from build123d import *

# Parameters (mm, degrees)
Y_KSEKLIK_EKSTR_ZYON3_DEPTH = 76
IZIM9_W                     = 50
IZIM9_H                     = 50
KES_EKSTR_ZYON2_DEPTH       = 72
RADYUS2_RADIUS              = 38
RADYUS2_LENGTH              = 18
IZIM10_R                    = 12.5
KES_EKSTR_ZYON3_DEPTH       = 260.686142434
FEDER1_REACH                = 253.207
IZIM11_WALL_W               = 579.380403386
IZIM11_WALL_H               = 22


with BuildPart() as part:
    # Çizim8 → Yükseklik-Ekstrüzyon3 (new body)
    with BuildSketch(Plane.XY):
        Polygon((-185.934081036, 55.935614824), (-109.934081036, 55.935614824), (-109.934081036, -16.064385176), (-241.934081036, -16.064385176), (-241.934081036, 1.935614824), (-185.934081036, 1.935614824), align=None)
    extrude(amount=Y_KSEKLIK_EKSTR_ZYON3_DEPTH)

    # Çizim9 → Kes-Ekstrüzyon2 (cut)
    with BuildSketch(Plane(origin=(0, 55.935614824, 0), x_dir=(1, 0, 0), z_dir=(0, 1, 0))):
        with Locations((-147.934081036, -38)):
            Rectangle(IZIM9_W, IZIM9_H)
    extrude(amount=-KES_EKSTR_ZYON2_DEPTH, mode=Mode.SUBTRACT)

    # Radyus2: full round fillet: the end face becomes a half cylinder, R = half its width
    radyus2_face = Plane((-241.934081036, -7.064385176, 38), x_dir=(0, 1, 0), z_dir=(-1, 0, 0))  # on the end face: x along it, z out of the body
    radyus2_slab = radyus2_face.offset(-RADYUS2_RADIUS / 2) * Box(RADYUS2_LENGTH, 2 * RADYUS2_RADIUS, RADYUS2_RADIUS, mode=Mode.PRIVATE)  # the body's end, R deep
    radyus2_round = Plane((-203.934081036, -7.064385176, 38), x_dir=(-1, 0, 0), z_dir=(0, 1, 0)) * Cylinder(RADYUS2_RADIUS, RADYUS2_LENGTH, mode=Mode.PRIVATE)  # its axis R under the face
    add(radyus2_slab - radyus2_round, mode=Mode.SUBTRACT)

    # Çizim10 → Kes-Ekstrüzyon3 (cut, through all)
    with BuildSketch(Plane.XY.offset(76)):
        with Locations((-147.934081036, 19.935614824)):
            Circle(IZIM10_R)
    extrude(amount=-KES_EKSTR_ZYON3_DEPTH, mode=Mode.SUBTRACT)

    # Çizim11 wall → Feder1 (add, up to next)
    with BuildSketch(Plane(origin=(-211.934081036, 28.935614824, 38), x_dir=(-0.693641687066, -0.720320213491, 0), z_dir=(0.720320213491, -0.693641687066, 0)), mode=Mode.PRIVATE) as feder1_sk1:
        Rectangle(IZIM11_WALL_W, IZIM11_WALL_H)
    feder1_tool1 = extrude(feder1_sk1.sketch, amount=FEDER1_REACH, mode=Mode.PRIVATE) - part.part
    add(feder1_tool1.solids().sort_by_distance((-211.934081036, 28.935614824, 38))[0])


solid = part.part
CAD build for the part. Positions are in the model's coordinates, mm. A direction names the side the tool comes from. Round coordinates to 2 decimals unless told otherwise and drop trailing zeros. Write each loop counter-clockwise with the first axis right and the second up, starting at its lowest first coordinate (ties: lowest second). Pieces come first, ordered by that corner, then holes. Notation, with made-up numbers: M -6.75,27 L 11.25,27 A17 ccw 11.25,43 Z; hole C 27,-20 d2. An arc over 180 degrees is marked long. Use a Markdown table: item, result. Add a question column.
1. Flat gauge pins, fed straight in: P1, Ø5, axis at x = -203, z = 41.5, coming from the +Y side; P2, Ø1.5, axis at x = -151, y = 48, coming from the -Z side; P3, Ø5, axis at y = -6.5, z = 60, coming from the -X side; P4, Ø10, axis at y = 24.5, z = 31, coming from the -X side. Where does each tip first touch, or does it go through?
2. Slice it at D-D on z = 64.5. Give the cut face in (x, y), then the cut area to 3 significant figures.
3. Slice it at A-A on z = 38. Give the cut face in (x, y).
4. Pull direction Y, two halves, no side cores. Call faces 1 (the face through (-211.57, 29.314, 37.846)), 2 (the face through (-136.01, 23.69, 6.59)), 3 (the face through (-185.934, 29, 62)): released by +Y, released by -Y, zero draft, split by the parting line, or undercut.
5. Slice it at B-B on y = 22. Give the cut face in (x, z), then the cut area to 3 significant figures.
6. Drill centre lines: probe 1 along Z at (x, y) = (-166, 30.5); probe 2 along X at (y, z) = (21.5, 54.5); probe 3 along X at (y, z) = (44, 71). Where is each one in solid material? Low to high.
7. 3-axis set-ups, long thin cutter, end or side, ignore diameter. For faces 4 (the face through (-201, 19, 27)), 5 (the face through (-201, 19, 49)), 6 (the face through (-172.934, 20, 38)), 7 (the face through (-208, 1.936, 54)), 8 (the face through (-148, 55.936, 12)): which of +Z, -Z, +X, -X, +Y, -Y reach the whole face in a straight line?
8. Slice it at C-C on y = 5. Give the cut face in (x, z).
Reply:
| question | item | result |
|---|---|---|
| 1 | P1 | stops at y = 40.81 |
| 1 | P2 | stops at z = 0 |
| 1 | P3 | stops at x = -236.55 |
| 1 | P4 | stops at x = -221.02 |
| 2 | outline | M -231.17,-16.06 L -109.93,-16.06 L -109.93,55.94 L -185.93,55.94 L -185.93,1.94 L -231.17,1.94 Z; hole C -147.93,19.94 d25 |
| 2 | area | 5,800 mm^2 |
| 3 | outline | M -241.93,-16.06 L -172.93,-16.06 L -172.93,55.94 L -185.93,55.94 L -237.93,1.94 L -241.93,1.94 Z; M -122.93,-16.06 L -109.93,-16.06 L -109.93,55.94 L -122.93,55.94 Z |
| 4 | face 1 | released by +Y |
| 4 | face 2 | undercut |
| 4 | face 3 | zero draft |
| 5 | outline | M -218.61,27 L -185.93,27 L -185.93,0 L -160.26,0 L -160.26,13 L -172.93,13 L -172.93,63 L -160.26,63 L -160.26,76 L -185.93,76 L -185.93,49 L -218.61,49 Z; M -135.61,0 L -109.93,0 L -109.93,76 L -135.61,76 L -135.61,63 L -122.93,63 L -122.93,13 L -135.61,13 Z |
| 5 | area | 3,350 mm^2 |
| 6 | probe 1 | z = 0 to 13, 63 to 76 |
| 6 | probe 2 | x = -185.93 to -172.93, -122.93 to -109.93 |
| 6 | probe 3 | x = -185.93 to -109.93 |
| 7 | face 4 | -Z, -X, +Y |
| 7 | face 5 | +Z, -X, +Y |
| 7 | face 6 | +Y, -Y |
| 7 | face 7 | -X, +Y |
| 7 | face 8 | +Z, -Z, +X, -X, +Y |
| 8 | outline | M -234.98,27 L -185.93,27 L -185.93,0 L -109.93,0 L -109.93,76 L -185.93,76 L -185.93,49 L -234.98,49 Z; hole M -172.93,13 L -122.93,13 L -122.93,63 L -172.93,63 Z |
